Can you work these out from the model? Positions are in its coordinate system, mm. A direction names the side the tool comes from. Give positions to 0.01 mm unless a question says otherwise; leave off trailing zeros. Order: outer loops, then holes, each group sorted by start corner. A loop starts at its lowest first (then second) coordinate and runs counter-clockwise, first axis right, second up. Notation, with made-up numbers: (35, -25.5) -> (76, -25.5) arc R11 cw to (76, -7.5) -> close; hole circle Ø2 at (-3, 11.25). An arc over 180 degrees is marked (long way). Answer as CSV lines item,"result".
```python
from build123d import *

# Parameters (mm, degrees)
F1_DEPTH = 50


with BuildPart() as f1:
    # F0 (on Front) → F1 (new body)
    with BuildSketch(Plane.XZ):
        with BuildLine():
            Line((-25, 124.041277), (0, 124.041277))
            Line((0, 124.041277), (0, 154.041277))
            Line((0, 154.041277), (-25, 154.041277))
            ThreePointArc((-25, 154.041277), (-26.464466, 150.505743), (-30, 149.041277))
            Line((-30, 149.041277), (-70, 149.041277))
            ThreePointArc((-70, 149.041277), (-73.535534, 150.505743), (-75, 154.041277))
            Line((-75, 154.041277), (-100, 154.041277))
            Line((-100, 154.041277), (-100, 124.041277))
            Line((-100, 124.041277), (-75, 124.041277))
            ThreePointArc((-75, 124.041277), (-73.535534, 127.57681), (-70, 129.041277))
            Line((-70, 129.041277), (-30, 129.041277))
            ThreePointArc((-30, 129.041277), (-26.464466, 127.57681), (-25, 124.041277))
        make_face()
        with BuildLine():
            Line((-25, 154.041277), (0, 154.041277))
            Line((0, 154.041277), (0, 184.041277))
            Line((0, 184.041277), (-25, 184.041277))
            ThreePointArc((-25, 184.041277), (-26.464466, 180.505743), (-30, 179.041277))
            Line((-30, 179.041277), (-70, 179.041277))
            ThreePointArc((-70, 179.041277), (-73.535534, 180.505743), (-75, 184.041277))
            Line((-75, 184.041277), (-100, 184.041277))
            Line((-100, 184.041277), (-100, 154.041277))
            Line((-100, 154.041277), (-75, 154.041277))
            ThreePointArc((-75, 154.041277), (-73.535534, 157.57681), (-70, 159.041277))
            Line((-70, 159.041277), (-30, 159.041277))
            ThreePointArc((-30, 159.041277), (-26.464466, 157.57681), (-25, 154.041277))
        make_face()
        with BuildLine():
            Line((-25, 184.041277), (0, 184.041277))
            Line((0, 184.041277), (0, 214))
            Line((0, 214), (-100, 214))
            Line((-100, 214), (-100, 184.041277))
            Line((-100, 184.041277), (-75, 184.041277))
            ThreePointArc((-75, 184.041277), (-73.535534, 187.57681), (-70, 189.041277))
            Line((-70, 189.041277), (-30, 189.041277))
            ThreePointArc((-30, 189.041277), (-26.464466, 187.57681), (-25, 184.041277))
        make_face()
        with BuildLine():
            Line((-25, 94.041277), (0, 94.041277))
            Line((0, 94.041277), (0, 124.041277))
            Line((0, 124.041277), (-25, 124.041277))
            ThreePointArc((-25, 124.041277), (-26.464466, 120.505743), (-30, 119.041277))
            Line((-30, 119.041277), (-70, 119.041277))
            ThreePointArc((-70, 119.041277), (-73.535534, 120.505743), (-75, 124.041277))
            Line((-75, 124.041277), (-100, 124.041277))
            Line((-100, 124.041277), (-100, 94.041277))
            Line((-100, 94.041277), (-75, 94.041277))
            ThreePointArc((-75, 94.041277), (-73.535534, 97.57681), (-70, 99.041277))
            Line((-70, 99.041277), (-30, 99.041277))
            ThreePointArc((-30, 99.041277), (-26.464466, 97.57681), (-25, 94.041277))
        make_face()
        with BuildLine():
            Line((-25, 64.041277), (0, 64.041277))
            Line((0, 64.041277), (0, 94.041277))
            Line((0, 94.041277), (-25, 94.041277))
            ThreePointArc((-25, 94.041277), (-26.464466, 90.505743), (-30, 89.041277))
            Line((-30, 89.041277), (-70, 89.041277))
            ThreePointArc((-70, 89.041277), (-73.535534, 90.505743), (-75, 94.041277))
            Line((-75, 94.041277), (-100, 94.041277))
            Line((-100, 94.041277), (-100, 64.041277))
            Line((-100, 64.041277), (-75, 64.041277))
            ThreePointArc((-75, 64.041277), (-73.535534, 67.57681), (-70, 69.041277))
            Line((-70, 69.041277), (-30, 69.041277))
            ThreePointArc((-30, 69.041277), (-26.464466, 67.57681), (-25, 64.041277))
        make_face()
        with BuildLine():
            Line((-25, 34.041277), (0, 34.041277))
            Line((0, 34.041277), (0, 64.041277))
            Line((0, 64.041277), (-25, 64.041277))
            ThreePointArc((-25, 64.041277), (-26.464466, 60.505743), (-30, 59.041277))
            Line((-30, 59.041277), (-70, 59.041277))
            ThreePointArc((-70, 59.041277), (-73.535534, 60.505743), (-75, 64.041277))
            Line((-75, 64.041277), (-100, 64.041277))
            Line((-100, 64.041277), (-100, 34.041277))
            Line((-100, 34.041277), (-75, 34.041277))
            ThreePointArc((-75, 34.041277), (-73.535534, 37.57681), (-70, 39.041277))
            Line((-70, 39.041277), (-30, 39.041277))
            ThreePointArc((-30, 39.041277), (-26.464466, 37.57681), (-25, 34.041277))
        make_face()
        with BuildLine():
            Line((-100, 0), (0, 0))
            Line((0, 0), (0, 34.041277))
            Line((0, 34.041277), (-25, 34.041277))
            ThreePointArc((-25, 34.041277), (-26.464466, 30.505743), (-30, 29.041277))
            Line((-30, 29.041277), (-70, 29.041277))
            ThreePointArc((-70, 29.041277), (-73.535534, 30.505743), (-75, 34.041277))
            Line((-75, 34.041277), (-100, 34.041277))
            Line((-100, 34.041277), (-100, 0))
        make_face()
    extrude(amount=F1_DEPTH)


solid = f1.part
```
Item 1: For pin 1 (20 mm diameter, centred on x = -49, y = -34.5, fed in from -Z), with a flat end and sliding along its axis, tell me the tip position at first contact or that it passes through.
Numbers:
pin 1,"stops at z = 0"
Item 2: For faces 1 (the flat face through (-51, -25, 0)), 2 (the flat face through (-50, -25, 99.041)), which set-ups out of +Z, -Z, +X, -X, +Y, -Y let a thin tool reach every point of the face, with its end or its side?
Numbers:
face 1,"-Z, +X, -X, +Y, -Y"
face 2,"+Y, -Y"
Item 3: We'd pull the mould along X, two halves only. Please class faces 3 (the flat face through (-100, -25, 108)), 4 (the flat face through (-50, -25, 69.041)), 5 (the flat face through (0, -25, 106)), 6 (the flat face through (-51, -50, 108)): released by +X, released by -X, zero draft, split by the parting line, or undercut.
Numbers:
face 3,"released by -X"
face 4,"undercut"
face 5,"released by +X"
face 6,"zero draft"
Item 4: Imagine slicing it at C-C, the plane y = -42. Give the number of separate pieces and of enclosed holes in the cut face, then the cut area to 3 significant figures.
Numbers:
separate pieces,"1"
enclosed holes,"6"
area,"18,500 mm²"
Item 5: Please list where these lines run through material, in increasing order: line 1 along X through (y, z) = (-31, 184); line 2 along X through (y, z) = (-30.5, 38.5).
Numbers:
line 1,"x = -100 to -75, -25 to 0"
line 2,"x = -100 to -72.26, -27.74 to 0"
Item 6: Imagine slicing it at A-A, the plane x = -48.5. Please give me the cut outline in (y, z).
Numbers:
outline,"(-50, 0) -> (0, 0) -> (0, 29.04) -> (-50, 29.04) -> close; (-50, 39.04) -> (0, 39.04) -> (0, 59.04) -> (-50, 59.04) -> close; (-50, 69.04) -> (0, 69.04) -> (0, 89.04) -> (-50, 89.04) -> close; (-50, 99.04) -> (0, 99.04) -> (0, 119.04) -> (-50, 119.04) -> close; (-50, 129.04) -> (0, 129.04) -> (0, 149.04) -> (-50, 149.04) -> close; (-50, 159.04) -> (0, 159.04) -> (0, 179.04) -> (-50, 179.04) -> close; (-50, 189.04) -> (0, 189.04) -> (0, 214) -> (-50, 214) -> close"
Item 7: Imagine slicing it at B-B, the plane z = 36. Please give me the cut outline in (x, y).
Numbers:
outline,"(-100, -50) -> (-74.6, -50) -> (-74.6, 0) -> (-100, 0) -> close; (-25.4, -50) -> (0, -50) -> (0, 0) -> (-25.4, 0) -> close"
